Verification items for the finished model (mm, model axes). Coordinates: 2 decimals unless noted, no trailing zeros. Write each loop counter-clockwise with the first axis right and the second up, starting at its lowest first coordinate (ties: lowest second). Pieces come first, ordered by that corner, then holes. Notation, with made-up numbers: M 75,-29.75 L 92,-29.75 A30 ccw 92,3.25 Z; hole C 7.25,8 d5. An arc over 180 degrees is marked long. One line per item, written item: value.
```python
from build123d import *

# Parameters (mm, degrees)
SKETCH1_W           = 11.675882566
SKETCH1_H           = 37.242609939
SKETCH1_H_2         = 37.242609938
BOSS_EXTRUDE1_DEPTH = 4


with BuildPart() as part:
    # Sketch1 → Boss-Extrude1 (new body)
    with BuildSketch(Plane.XY):
        Polygon((6.4, 64.343953413), (-11.2, 64.343953413), (-11.2, 60.343953413), (-28.8, 60.343953413), (-28.8, 64.343953413), (-46.4, 64.343953413), (-46.4, 60.343953413), (-64, 60.343953413), (-64, -21.996281697), (-68, -21.996281697), (-68, -41.996281697), (-64, -41.996281697), (-64, -81.996281697), (-68, -81.996281697), (-68, -101.996281697), (-64, -101.996281697), (-64, -141.996281697), (-68, -141.996281697), (-68, -161.996281697), (-64, -161.996281697), (-64, -201.996281697), (-68, -201.996281697), (-68, -221.996281697), (-64, -221.996281697), (-64, -226.996281697), (24, -226.996281697), (24, -221.996281697), (28, -221.996281697), (28, -201.996281697), (24, -201.996281697), (24, -161.996281697), (28, -161.996281697), (28, -141.996281697), (24, -141.996281697), (24, -101.996281697), (28, -101.996281697), (28, -81.996281697), (24, -81.996281697), (24, -41.996281697), (28, -41.996281697), (28, -21.996281697), (24, -21.996281697), (24, 60.343953413), (6.4, 60.343953413), align=None)
        with Locations((-32.17836291, -181.887864713)):
            Rectangle(SKETCH1_W, SKETCH1_H, mode=Mode.SUBTRACT)
        with Locations((-7.82163709, 18.983890438)):
            Rectangle(SKETCH1_W, SKETCH1_H, mode=Mode.SUBTRACT)
        with Locations((-7.82163709, -43.686747162)):
            Rectangle(SKETCH1_W, SKETCH1_H, mode=Mode.SUBTRACT)
        with Locations((-7.82163709, -115.460501141)):
            Rectangle(SKETCH1_W, SKETCH1_H_2, mode=Mode.SUBTRACT)
        with Locations((-7.82163709, -181.887864713)):
            Rectangle(SKETCH1_W, SKETCH1_H, mode=Mode.SUBTRACT)
        with Locations((-32.17836291, -115.460501141)):
            Rectangle(SKETCH1_W, SKETCH1_H_2, mode=Mode.SUBTRACT)
        with Locations((-32.17836291, -43.686747162)):
            Rectangle(SKETCH1_W, SKETCH1_H, mode=Mode.SUBTRACT)
        with Locations((-32.17836291, 18.983890438)):
            Rectangle(SKETCH1_W, SKETCH1_H, mode=Mode.SUBTRACT)
    extrude(amount=BOSS_EXTRUDE1_DEPTH)


solid = part.part
```
Item 1: Cross-section at C-C, the plane z = 1.4. Give the number of separate pieces and of enclosed holes in the cut face, and give its area (3 significant figures).
The answers:
separate pieces: 1
enclosed holes: 8
area: 22,600 mm²
Item 2: Scan lines: line 1 (X direction, y = -39, z = 0.85); line 2 (X direction, y = -175, z = 3.45); line 3 (Y direction, x = -28.5, z = 2.15). Record each from-to range of solid material in increasing order.
The answers:
line 1: x = -68 to -38.02, -26.34 to -13.66, -1.98 to 28
line 2: x = -64 to -38.02, -26.34 to -13.66, -1.98 to 24
line 3: y = -227 to -200.51, -163.27 to -134.08, -96.84 to -62.31, -25.07 to 0.36, 37.61 to 60.34
Item 3: Cross-section at D-D, the plane y = -10. Enter the section's corners in (x, z).
The answers:
outline: M -64,0 L 24,0 L 24,4 L -64,4 Z
Item 4: Cross-section at A-A, the plane y = -106. Enter the section's corners in (x, z), and give its area (3 significant figures).
The answers:
outline: M -64,0 L -38.02,0 L -38.02,4 L -64,4 Z; M -26.34,0 L -13.66,0 L -13.66,4 L -26.34,4 Z; M -1.98,0 L 24,0 L 24,4 L -1.98,4 Z
area: 259 mm²
Item 5: Cross-section at B-B, the plane x = -6. Enter the section's corners in (y, z), and give its area (3 significant figures).
The answers:
outline: M -227,0 L -200.51,0 L -200.51,4 L -227,4 Z; M -163.27,0 L -134.08,0 L -134.08,4 L -163.27,4 Z; M -96.84,0 L -62.31,0 L -62.31,4 L -96.84,4 Z; M -25.07,0 L 0.36,0 L 0.36,4 L -25.07,4 Z; M 37.61,0 L 64.34,0 L 64.34,4 L 37.61,4 Z
area: 569 mm²
Item 6: Go/stop test with flat-tipped pins: P1, Ø1.2, axis at y = -116.5, z = 1.5, coming from the -X side; P2, Ø1, axis at y = -53.5, z = 1.5, coming from the +X side; P3, Ø1, axis at x = -17, z = 1.5, coming from the +Y side. Record where each tip stops, or that it passes through.
The answers:
P1: stops at x = -64
P2: stops at x = 24
P3: stops at y = 60.34
